CAD build for the part. Positions are in the model's coordinates, mm. A direction names the side the tool comes from. Round coordinates to 2 decimals unless told otherwise and drop trailing zeros. Loops run counter-clockwise (first coordinate to the right, second up) from the corner with the lowest first, then second, coordinate; pieces in that order, holes last. Notation, with made-up numbers: M 51.25,32.25 L 97.25,32.25 A23 cw 97.25,41.25 Z; hole C 88.5,-27.5 d1. An arc over 180 degrees is marked long. Use one line per item in the form item = value.
from build123d import *

# Parameters (mm, degrees)
F1_DEPTH = 25.4
F2_R     = 1.5748


with BuildPart() as f1:
    # F0 (on Top) → F1 (new body)
    with BuildSketch(Plane.XY):
        with BuildLine():
            Line((-41.113433, 16.30855), (-41.113433, -15.44145))
            Line((-41.113433, -15.44145), (9.686567, -15.44145))
            Line((9.686567, -15.44145), (16.421759, -22.176642))
            Line((16.421759, -22.176642), (54.521759, -22.176642))
            ThreePointArc((54.521759, -22.176642), (66.836567, 0.43355), (54.521759, 23.043742))
            Line((54.521759, 23.043742), (16.421759, 23.043742))
            Line((16.421759, 23.043742), (9.686567, 16.30855))
            Line((9.686567, 16.30855), (-41.113433, 16.30855))
        make_face()
    extrude(amount=F1_DEPTH)

    # F2
    f2_edges = [f1.edges().sort_by_distance(p)[0] for p in [
        (35.471759, 23.043742, 25.4),
        (13.054163, 19.676146, 25.4),
        (-15.713433, 16.30855, 25.4),
        (-41.113433, 0.43355, 25.4),
        (-15.713433, -15.44145, 25.4),
        (13.054163, -18.809046, 25.4),
        (35.471759, -22.176642, 25.4),
        (66.836567, 0.43355, 25.4),
    ]]
    fillet(f2_edges, radius=F2_R)


solid = f1.part
1. Drop flat-ended pins along their axis: P1, Ø5, axis at y = 2.5, z = 14, coming from the +X side; P2, Ø3, axis at y = 4.5, z = 19.5, coming from the +X side; P3, Ø6, axis at x = -8, z = 9, coming from the +Y side. Give the stop position or say it passes through.
Completed:
P1 = 66.84
P2 = 66.71
P3 = 16.31
2. Cut at A-A on z = 10. Write the cut outline in (x, y), and give its area (3 significant figures).
Completed:
outline = M -41.11,-15.44 L 9.69,-15.44 L 16.42,-22.18 L 54.52,-22.18 A26.91 ccw 54.52,23.04 L 16.42,23.04 L 9.69,16.31 L -41.11,16.31 Z
area = 3,990 mm2
3. Cut at B-B on x = -4.5. Write the cut outline in (y, z), and give its area (3 significant figures).
Completed:
outline = M -15.44,0 L 16.31,0 L 16.31,23.83 A1.57 ccw 14.73,25.4 L -13.87,25.4 A1.57 ccw -15.44,23.83 Z
area = 805 mm2
4. Tool access for faces 1 (the face through (-16, -15.441, 12)), 2 (the face through (-15, 16.309, 12)), 3 (the face through (13.191, -18.311, 24.926)): list every direction of +Z, -Z, +X, -X, +Y, -Y with a clear straight run to the whole face (end or side of a thin tool).
Completed:
face_1 = +Z, -Z, -X, -Y
face_2 = +Z, -Z, -X, +Y
face_3 = +Z, -X, -Y
5. Probe line 1 along Y through (x, z) = (-5.5, 15.75); line 2 along X through (y, z) = (9.5, 10.5); line 3 along X through (y, z) = (15, 3.25). List the from-to ranges inside material, lowest first. Write a range as from..to.
Completed:
line_1 = -15.44..16.31
line_2 = -41.11..65.26
line_3 = -41.11..62.55
